Check sheet for the modelled part. Datum: model origin and axes. Units: mm. Give positions to 0.01 mm unless a question says otherwise; leave off trailing zeros. Write each loop counter-clockwise with the first axis right and the second up, starting at its lowest first coordinate (ties: lowest second). Pieces come first, ordered by that corner, then holes. Notation, with made-up numbers: (45.5, 36) -> (62.5, 36) arc R10 cw to (62.5, 50) -> close; hole circle Ø3 at (0.5, 72.25). An arc over 180 degrees is marked (long way). Use a Markdown table: item, result. Add a question column.
1. Cross-section at A-A (z = 0.65). Enter the section's corners in (x, y).
2. Cross-section at B-B (y = -12). Enter the section's corners in (x, z), then the cut area to 3 significant figures.
3. Cross-section at C-C (x = -16). Enter the section's corners in (y, z), then the cut area to 3 significant figures.
4. Scan lines: probe 1 along X at (y, z) = (-2, 0.3); probe 2 along Y at (x, z) = (-4.5, 0.3); probe 3 along X at (y, z) = (-11, 0.15). Record each from-to range of solid material in increasing order. Write a range as [from, to].
5. Release check for a two-part mould opening along Y. For faces 1 (the flat face through (-19.6, 0, 0.5)), 2 (the flat face through (0, 0, 1)), 3 (the flat face through (19.6, 0, 0.5)), 4 (the cylindrical face through (-0.408, -19.996, 0.493)) record: released by +Y, released by -Y, zero draft, split by the parting line, or undercut.
from build123d import *

# Parameters (mm, degrees)
SKETCH1_R           = 20
BOSS_EXTRUDE1_DEPTH = 1
CUT_EXTRUDE1_DEPTH  = 1
CIRPATTERN1_COUNT   = 2


with BuildPart() as part:
    # Sketch1 → Boss-Extrude1 (new body)
    with BuildSketch(Plane.XY):
        Circle(SKETCH1_R)
    extrude(amount=BOSS_EXTRUDE1_DEPTH)

    # Sketch2 → Cut-Extrude1 (cut)
    with BuildSketch(Plane.XY.offset(1)):
        with BuildLine():
            Line((-19.867309833, 2.3), (-19.8, 2.3))
            ThreePointArc((-19.8, 2.3), (-19.658578644, 2.241421356), (-19.6, 2.1))
            Line((-19.6, 2.1), (-19.6, -2.1))
            ThreePointArc((-19.6, -2.1), (-19.658578644, -2.241421356), (-19.8, -2.3))
            Line((-19.8, -2.3), (-19.867309833, -2.3))
            ThreePointArc((-19.867309833, -2.3), (-20, 0), (-19.867309833, 2.3))
        make_face()
    cut_extrude1 = extrude(amount=-CUT_EXTRUDE1_DEPTH, mode=Mode.SUBTRACT)

    # CirPattern1: Cut-Extrude1 ×2 about axis
    cirpattern1_axis = Axis((0, 0, 0), (0, 0, 1))
    for i in range(1, CIRPATTERN1_COUNT):
        add(cut_extrude1.rotate(cirpattern1_axis, i * 360 / CIRPATTERN1_COUNT), mode=Mode.SUBTRACT)


solid = part.part
Worked answers:
| question | item | result |
|---|---|---|
| 1 | outline | (-19.87, -2.3) arc R20 ccw to (19.87, -2.3) -> (19.8, -2.3) arc R0.2 cw to (19.6, -2.1) -> (19.6, 2.1) arc R0.2 cw to (19.8, 2.3) -> (19.87, 2.3) arc R20 ccw to (-19.87, 2.3) -> (-19.8, 2.3) arc R0.2 cw to (-19.6, 2.1) -> (-19.6, -2.1) arc R0.2 cw to (-19.8, -2.3) -> close |
| 2 | outline | (-16, 0) -> (16, 0) -> (16, 1) -> (-16, 1) -> close |
| 2 | area | 32.0 mm² |
| 3 | outline | (-12, 0) -> (12, 0) -> (12, 1) -> (-12, 1) -> close |
| 3 | area | 24.0 mm² |
| 4 | probe 1 | x = [-19.6, 19.6] |
| 4 | probe 2 | y = [-19.49, 19.49] |
| 4 | probe 3 | x = [-16.7, 16.7] |
| 5 | face 1 | undercut |
| 5 | face 2 | zero draft |
| 5 | face 3 | undercut |
| 5 | face 4 | released by -Y |
